The listing builds one solid part. Answer for the finished solid, in the listing's coordinates (mm). Give positions to 0.01 mm unless a question says otherwise; leave off trailing zeros. Order: outer loops, then holes, each group sorted by start corner. A loop starts at its lowest first (then second) coordinate and runs counter-clockwise, first axis right, second up. Notation, with made-up numbers: (-27, 36.5) - (-20, 36.5) arc R16 ccw to (-20, 65.5) - close; hole circle Ø9 at (48.25, 88). An arc over 180 degrees is marked (long way). Answer in a Markdown table with one row per item.
from build123d import *

# Parameters (mm, degrees)
F1_DEPTH = 330.2
F3_DEPTH = 84.1385
F4_R     = 11.1125
F5_DEPTH = 84.1385


with BuildPart() as f1:
    # F0 (on Front) → F1 (new body)
    with BuildSketch(Plane.XZ):
        with BuildLine():
            ThreePointArc((-43.65625, 8.362675), (0, 44.45), (43.65625, 8.362675))
            Line((43.65625, 8.362675), (43.65625, 71.925314))
            ThreePointArc((43.65625, 71.925314), (0, 84.1375), (-43.65625, 71.925314))
            Line((-43.65625, 71.925314), (-43.65625, 8.362675))
        make_face()
    extrude(amount=-F1_DEPTH)

    # F2 (on Top) → F3 (cut, through all)
    with BuildSketch(Plane.XY):
        with BuildLine():
            Line((-43.65625, 330.2), (-43.65625, 292.1))
            ThreePointArc((-43.65625, 292.1), (-28.971875, 319.335547), (0, 330.2))
            Line((0, 330.2), (-43.65625, 330.2))
        make_face()
        with BuildLine():
            Line((43.65625, 330.2), (0, 330.2))
            ThreePointArc((0, 330.2), (28.971875, 319.335547), (43.65625, 292.1))
            Line((43.65625, 292.1), (43.65625, 330.2))
        make_face()
    extrude(amount=F3_DEPTH, mode=Mode.SUBTRACT)

    # F4 (on Top) → F5 (cut, through all)
    with BuildSketch(Plane.XY):
        with Locations((0, 241.3)):
            Circle(F4_R)
        with Locations((0, 38.1)):
            Circle(F4_R)
    extrude(amount=F5_DEPTH, mode=Mode.SUBTRACT)


solid = f1.part
Item 1: Determine the mould class of faces 1 (the face through (0.643, 162.789, 84.135)), 2 (the face through (-1, 0, 55)), 3 (the face through (43.656, 144, 40)), 4 (the face through (-2.41, 27.25, 63.3)) for opening direction X: pulls with the +X half, pulls with the -X half, needs draft (parallel to the pull), parting line crosses it, or undercut.
Answer block:
| item | result |
|---|---|
| face 1 | parting line crosses it |
| face 2 | needs draft |
| face 3 | pulls with the +X half |
| face 4 | undercut |
Item 2: Find section A-A on z = 34.5. Write down the section's boundary in (x, y).
Answer block:
| item | result |
|---|---|
| outline | (-43.66, 0) - (-28.03, 0) - (-28.03, 320.14) arc R44.06 ccw to (-43.66, 292.1) - close; (28.03, 0) - (43.66, 0) - (43.66, 292.1) arc R44.06 ccw to (28.03, 320.14) - close |
Item 3: Find section D-D on x = 21.5. Write down the section's boundary in (y, z).
Answer block:
| item | result |
|---|---|
| outline | (0, 38.9) - (324.6, 38.9) - (324.6, 81.34) - (0, 81.34) - close |
Item 4: Each of these flat-tipped pins is pushed along its axis until it touches: P1, Ø12, axis at x = 22, z = 63.5, coming from the -Y side; P2, Ø8, axis at x = -8.5, y = 286.5, coming from the +Z side; P3, Ø5, axis at x = -4, z = 76.5, coming from the +Y side; P4, Ø6, axis at x = -30, y = 78.5, coming from the +Z side. Where does it stop, or does it pass through?
Answer block:
| item | result |
|---|---|
| P1 | y = 0 |
| P2 | z = 84.02 |
| P3 | y = 330.17 |
| P4 | z = 79.69 |
Item 5: Consider line 1 (Y direction, x = 0, z = 68); line 2 (X direction, y = 241.3, z = 53); line 3 (Z direction, x = -2, y = 110). Determine where each line is inside the solid, lowest interval first.
Answer block:
| item | result |
|---|---|
| line 1 | 0 to 26.99, 49.21 to 230.19, 252.41 to 330.2 |
| line 2 | -43.66 to -11.11, 11.11 to 43.66 |
| line 3 | 44.4 to 84.11 |
